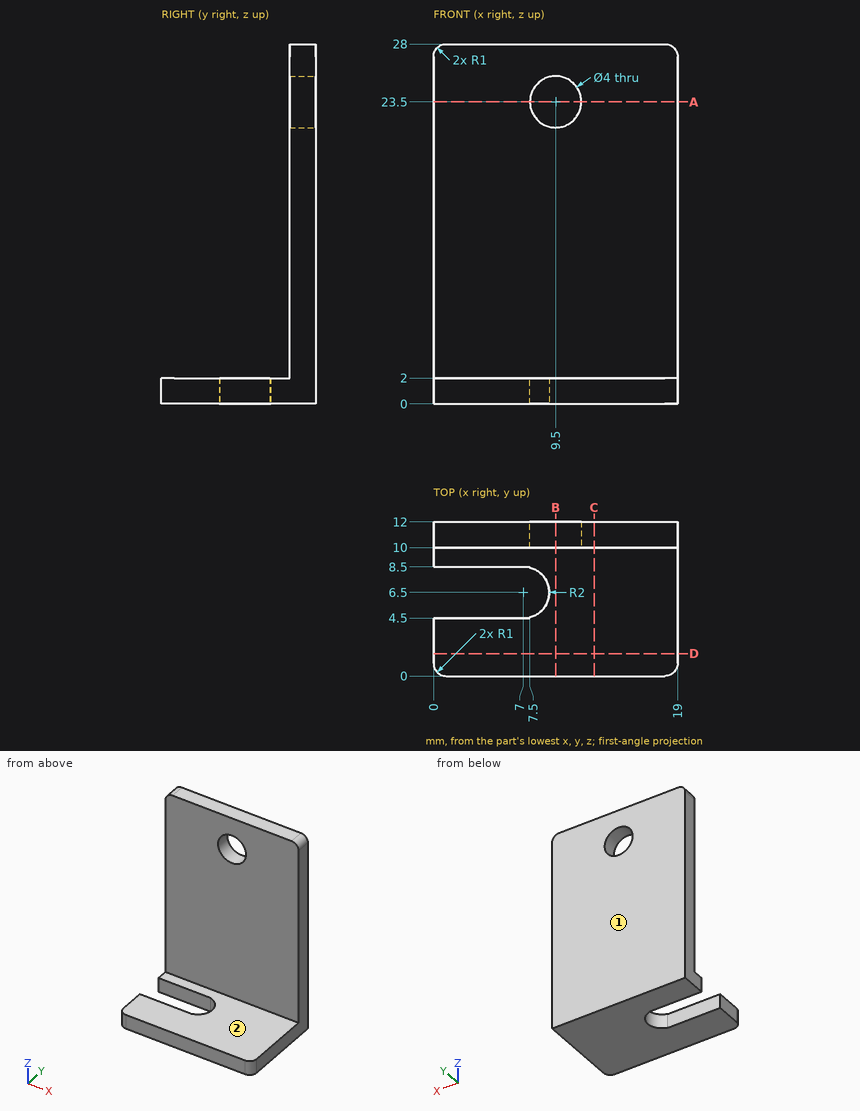
Input: dimensioned drawing with shaded views. Units: mm. Origin: part minimum x, y, z. A direction names the side the tool comes from. Coordinates: 2 decimals unless noted, no trailing zeros. Loops run counter-clockwise (first coordinate to the right, second up) from the corner with the lowest first, then second, coordinate; pieces in that order, holes last. Notation, with made-up numbers: M -29.5,88.5 L -11.5,88.5 A19 cw -11.5,108.5 Z; hole C -16.5,72 d4. An arc over 180 degrees is marked long. One line per item, written item: value.
(1) Line query: line 1 along Z through (x, y) = (9.5, 11.55); line 2 along Z through (x, y) = (2.25, 1); line 3 along Y through (x, z) = (17.5, 26). Output: solid intervals per line, ascending. Write a range as from..to.
Filled in:
line 1: 0..21.5, 25.5..28
line 2: 0..2
line 3: 10..12
(2) Section A-A (z = 23.5). Output: boundary loops of the cut face in (x, y).
Filled in:
outline: M 0,10 L 7.5,10 L 7.5,12 L 0,12 Z; M 11.5,10 L 19,10 L 19,12 L 11.5,12 Z
(3) Reachability of the marked faces 1 and 2 from +Z, -Z, +X, -X, +Y, -Y: full face, straight path, thin tool, end or side. Return the list, or none.
Filled in:
face 1: +Z, -Z, +X, -X, +Y
face 2: +Z, +X, -X, -Y
(4) Section C-C (x = 12.5). Output: boundary loops of the cut face in (y, z).
Filled in:
outline: M 0,0 L 12,0 L 12,28 L 10,28 L 10,2 L 0,2 Z
(5) Section B-B (x = 9.5). Output: boundary loops of the cut face in (y, z).
Filled in:
outline: M 0,0 L 12,0 L 12,21.5 L 10,21.5 L 10,2 L 0,2 Z; M 10,25.5 L 12,25.5 L 12,28 L 10,28 Z
(6) Section D-D (y = 1.75). Output: boundary loops of the cut face in (x, z).
Filled in:
outline: M 0,0 L 19,0 L 19,2 L 0,2 Z
(7) Pin query (flat end, axial travel): pin 1 (4.5 mm diameter, centred on x = 9.5, z = 23.5, fed in from -Y); pin 2 (3 mm diameter, centred on x = 8.5, y = 6, fed in from +Z); pin 3 (3 mm diameter, centred on y = 8, z = 5.5, fed in from +X). Return the tip coordinate at first contact, or that it passes through.
Filled in:
pin 1: y = 10
pin 2: z = 2
pin 3: through
